Source: three-view drawing plus pictorial views. Frame: mm from the lowest corner of the part. A direction names the side the tool comes from. Give positions to 0.01 mm unless a question says otherwise; leave off trailing zeros. Loops run counter-clockwise (first coordinate to the right, second up) from the corner with the lowest first, then second, coordinate; pieces in that order, holes last. Notation, with made-up numbers: (17.25, 68) - (39.25, 68) arc R9 cw to (39.25, 80) - close; hole circle Ø6 at (16, 0.5). An arc over 180 degrees is marked (long way). Write each question's results on one line, items separated by ' | '. Start each with the question number.
(1) Cut plane C-C on z = 9.75. Return the cut outline in (x, y).
(2) Pull-direction query (Z, two-part tool) for the marked faces 4, 5 and 6; classes: pulls with the +Z half, pulls with the -Z half, needs draft (parallel to the pull), parting line crosses it, or undercut.
(3) Reachability of the marked faces 1, 2 and 3 from +Z, -Z, +X, -X, +Y, -Y: full face, straight path, thin tool, end or side. Return the list, or none.
(4) Material intervals for line 1 along Z through (x, y) = (25.4, 22.75); line 2 along X through (y, z) = (8.5, 2.25); line 3 along Y through (x, z) = (16, 13.25), sorted ascending. Write a range as [from, to].
(5) Cut plane B-B on y = 3.75. Return the cut outline in (x, z).
(6) Cut plane D-D on x = 9. Return the cut outline in (y, z).
(7) Contact query for flat-ended pins moving along their axis: pin 1 (1.5 mm diameter, centred on y = 19, z = 21.5, fed in from +X); pin 2 (4 mm diameter, centred on x = 29.5, z = 18.5, fed in from -Y); pin 3 (6.5 mm diameter, centred on y = 6, z = 7, fed in from +X). Output: stop coordinate, or through.
(8) Cut plane A-A on x = 25.4. Return the cut outline in (y, z).
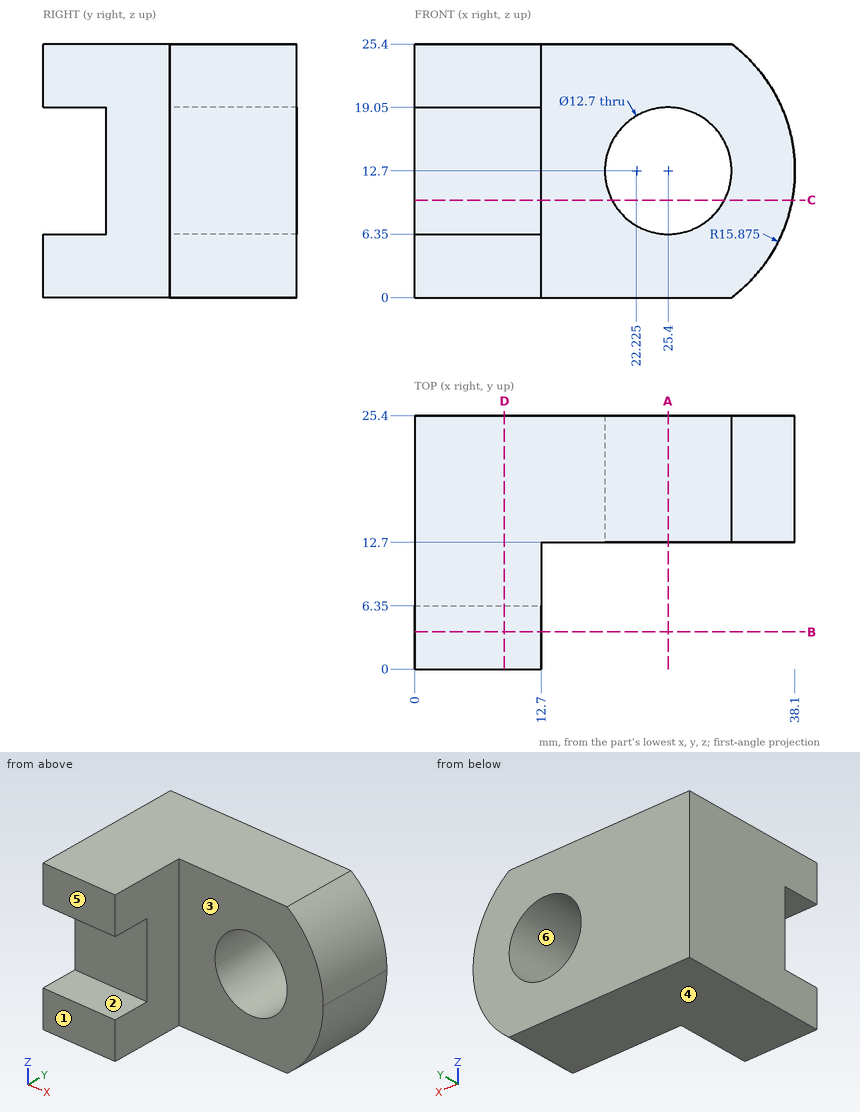
Ans:
1) outline: (0, 6.35) - (12.7, 6.35) - (12.7, 12.7) - (19.78, 12.7) - (19.78, 25.4) - (0, 25.4) - close; (31.02, 12.7) - (37.82, 12.7) - (37.82, 25.4) - (31.02, 25.4) - close
2) face 4: pulls with the -Z half | face 5: needs draft | face 6: undercut
3) face 1: +Z, -Z, +X, -X, -Y | face 2: +X, -X, -Y | face 3: +Z, -Z, +X, -Y
4) line 1: [0, 6.35], [19.05, 25.4] | line 2: [0, 12.7] | line 3: [12.7, 25.4]
5) outline: (0, 0) - (12.7, 0) - (12.7, 6.35) - (0, 6.35) - close; (0, 19.05) - (12.7, 19.05) - (12.7, 25.4) - (0, 25.4) - close
6) outline: (0, 0) - (25.4, 0) - (25.4, 25.4) - (0, 25.4) - (0, 19.05) - (6.35, 19.05) - (6.35, 6.35) - (0, 6.35) - close
7) pin 1: x = 35.91 | pin 2: y = 12.7 | pin 3: x = 12.7
8) outline: (12.7, 0) - (25.4, 0) - (25.4, 6.35) - (12.7, 6.35) - close; (12.7, 19.05) - (25.4, 19.05) - (25.4, 25.4) - (12.7, 25.4) - close
